Autodesk Inventor part; units mm, degrees
ref_plane "РабПлоскость2" through (-464.2239, 154.5996, -124.0538) normal (0, 1, 0) x (0, 0, 1)
ref_plane "YZ Plane" through (0, 0, 0) normal (1, 0, 0) x (0, 1, 0)
ref_plane "XZ Plane" through (0, 0, 0) normal (0, 1, 0) x (-1, 0, 0)
ref_plane "РабПлоскость1" through (-329.2239, 210.3045, -11.0538) normal (0, -1, 0) x (1, 0, 0)
sketch "Эскиз1" plane through (-329.2239, 210.3045, -11.0538) normal (0, -1, 0) x (1, 0, 0)
  line L0 (-46.5606, -73) -> (-52.5606, -73)
  line L1 (-52.5606, -73) -> (-52.5606, -43)
  line L2 (-52.5606, -43) -> (-46.5606, -43)
  line L3 (-46.5606, -43) -> (-46.5606, -73)
  line L4 (-23.55, -78) -> (-51.55, -78)
  point P0 (329.2239, 11.0538)
  dimension "d0" = 6
  dimension "d1" = 30
  dimension "d2" = 5
ref_plane "РабПлоскость2" through (-464.2239, 154.5996, -124.0538) normal (0, 1, 0) x (0, 0, 1)
extrude "Выдавливание1" add sketch "Эскиз1" along normal up to surface (55.705 mm away)
sketch "Эскиз2" plane through (-375.7846, 210.3045, -54.0538) normal (1, 0, 0) x (0, 0, -1)
  line L0 (0, -55.705) -> (30, -55.705)
  line L1 (30, -55.705) -> (23, -55.705)
  line L2 (23, -55.705) -> (23, -60.705)
  line L3 (23, -60.705) -> (30, -60.705)
  line L4 (30, -60.705) -> (30, -55.705)
  line L5 (0, -55.705) -> (7, -55.705)
  line L6 (7, -55.705) -> (7, -60.705)
  line L7 (7, -60.705) -> (0, -60.705)
  line L8 (0, -60.705) -> (0, -55.705)
  line L9 (18.25, -53.705) -> (11.75, -53.705)
  line L10 (11.75, -53.705) -> (11.75, -50.705)
  line L11 (11.75, -50.705) -> (18.25, -50.705)
  line L12 (18.25, -50.705) -> (18.25, -53.705)
  line L13 (13.25, -46.5052) -> (16.75, -46.5052)
  line L14 (16.75, -46.5052) -> (16.75, -57.9047)
  line L15 (16.75, -57.9047) -> (13.25, -57.9047)
  line L16 (13.25, -57.9047) -> (13.25, -46.5052)
  line L17 (13.25, -46.5052) -> (16.75, -57.9047) construction
  line L18 (16.75, -46.5052) -> (13.25, -57.9047) construction
  line L19 (30, 0) -> (30, -55.705)
  line L20 (30, -27.8525) -> (0, -27.8525)
  line L21 (0, 0) -> (0, -55.705)
  line L22 (30, 0) -> (23, 0)
  line L23 (23, 0) -> (23, 5)
  line L24 (23, 5) -> (30, 5)
  line L25 (30, 5) -> (30, 0)
  line L26 (0, 0) -> (7, 0)
  line L27 (7, 0) -> (7, 5)
  line L28 (7, 5) -> (0, 5)
  line L29 (0, 5) -> (0, 0)
  line L30 (18.25, -2) -> (11.75, -2)
  line L31 (11.75, -2) -> (11.75, -5)
  line L32 (11.75, -5) -> (18.25, -5)
  line L33 (18.25, -5) -> (18.25, -2)
  line L34 (13.25, -9.1998) -> (16.75, -9.1998)
  line L35 (16.75, -9.1998) -> (16.75, 2.1998)
  line L36 (16.75, 2.1998) -> (13.25, 2.1998)
  line L37 (13.25, 2.1998) -> (13.25, -9.1998)
  line L38 (13.25, -9.1998) -> (16.75, 2.1998) construction
  line L39 (16.75, -9.1998) -> (13.25, 2.1998) construction
  point P0 (-54.0538, -210.3045)
  point P1 (15, -52.205)
  point P2 (7, -55.705)
  point P3 (23, -55.705)
  point P4 (16.75, -53.705)
  point P5 (16.75, -50.705)
  point P6 (13.25, -50.705)
  point P7 (13.25, -53.705)
  point P8 (15, -3.5)
  point P9 (16.75, -5)
  point P10 (16.75, -2)
  point P11 (13.25, -2)
  point P12 (13.25, -5)
  dimension "d2" = 5
  dimension "d13" = 6.5
  dimension "d14" = 3
  dimension "d15" = 5
  dimension "d16" = 7
  dimension "d17" = 4.75
  dimension "d18" = 2
  dimension "d19" = 3.5
  dimension "d20" = 3.25
  dimension "d23" = 5
  dimension "d24" = 7
  dimension "d25" = 7
extrude "Выдавливание2" add sketch "Эскиз2" against normal blind 6 contours L0 L6 L7 L8 | L4 L3 L2 L0 | L22 L23 L24 L25 | L29 L28 L27 L26
sketch "Эскиз3" plane through (-375.7846, 154.5996, -84.0538) normal (1, 0, 0) x (0, 0, -1)
  point P0 (-84.0538, -154.5996)
extrude "Выдавливание3" cut sketch "Эскиз2" against normal blind 6 contours L16 L9 L14 L0 | L0 L14 L15 L16 | L16 L11 L14 L9 | L9 L10 L11 L16 | L14 L11 L12 L9 | L16 L13 L14 L11 | L33 L32 L35 L30 | L35 L32 L37 L30 | L30 L37 L36 L35 | L37 L32 L31 L30 | L35 L34 L37 L32
properties part number "стенка 2"
For this review, take the finished solid that the model builds, in its own axes (mm). A direction names the side the tool comes from. Give positions to 0.01 mm unless a question says otherwise; leave off trailing zeros. Loops run counter-clockwise (first coordinate to the right, second up) from the corner with the lowest first, then second, coordinate; pieces in that order, holes last. Notation, with made-up numbers: (16, 80) - (24, 80) arc R25 ccw to (24, 119) - close; hole circle Ø11 at (-26, 48). An arc over 180 degrees is marked (long way). Write each question's results on one line, items separated by ' | '.
(1) Take a section at A-A (y = 154). Give the boundary of the cut face in (x, z).
Conclusion:
outline: (-381.78, -84.05) - (-375.78, -84.05) - (-375.78, -77.05) - (-381.78, -77.05) - close; (-381.78, -61.05) - (-375.78, -61.05) - (-375.78, -54.05) - (-381.78, -54.05) - close
(2) For pin 1 Ø0.8 at (x, z) = (-378.5, -71.5) entering from +Y; pin 2 Ø1.6 at (x, z) = (-378, -71.5) entering from -Y, all flat-tipped, find the tip position at first contact; note any pin that passes through.
Conclusion:
pin 1: y = 210.3 | pin 2: y = 154.6
(3) For faces 1 (the flat face through (-379, 183, -84.054)), 2 (the flat face through (-379, 208.304, -67)), 3 (the flat face through (-379, 154.6, -64)), 4 (the flat face through (-379, 209, -70.804)), 5 (the flat face through (-379, 183, -54.054)), list the 3-axis set-ups (+Z, -Z, +X, -X, +Y, -Y) from which the entire face can be reached by the end or side of a thin tool; tool diameter is ignored.
Conclusion:
face 1: -Z, +X, -X, +Y, -Y | face 2: +X, -X | face 3: +X, -X, -Y | face 4: +X, -X, +Y | face 5: +Z, +X, -X, +Y, -Y
(4) For line 1 along Y through (x, z) = (-380, -67); line 2 along Z through (x, y) = (-380.5, 157.5); line 3 along Z through (x, y) = (-381.5, 212), list the stretches that pass through material, from the lowest coordinate up.
Conclusion:
line 1: 154.6 to 156.6, 159.6 to 205.3, 208.3 to 210.3 | line 2: -84.05 to -72.3, -65.8 to -54.05 | line 3: -84.05 to -77.05, -61.05 to -54.05
(5) Take a section at B-B (y = 206). Give the boundary of the cut face in (x, z), then the cut area to 3 significant figures.
Conclusion:
outline: (-381.78, -84.05) - (-375.78, -84.05) - (-375.78, -72.3) - (-381.78, -72.3) - close; (-381.78, -65.8) - (-375.78, -65.8) - (-375.78, -54.05) - (-381.78, -54.05) - close | area: 141 mm^2
(6) Take a section at C-C (z = -65). Give the boundary of the cut face in (x, y), then the cut area to 3 significant figures.
Conclusion:
outline: (-381.78, 154.6) - (-375.78, 154.6) - (-375.78, 210.3) - (-381.78, 210.3) - close | area: 334 mm^2
(7) Draft analysis for pull direction Y (two halves, no side actions). For faces 6 (the flat face through (-379, 210.304, -74)), 7 (the flat face through (-379, 149.6, -58)), 8 (the flat face through (-379, 205.304, -72)), state which applies: +Y half, -Y half, draft (parallel to the pull), parting line (faces both ways), or undercut.
Conclusion:
face 6: +Y half | face 7: -Y half | face 8: undercut
